Here's how the part is built. I have some questions about the finished solid (model axes, mm). Round coordinates to 2 decimals unless told otherwise and drop trailing zeros. Loops run counter-clockwise (first coordinate to the right, second up) from the corner with the lowest first, then second, coordinate; pieces in that order, holes last. Notation, with made-up numbers: M 68.25,49.25 L 124.25,49.25 A19 ccw 124.25,60.25 Z; hole C 18.25,83 d6. An arc over 180 degrees is marked long. One line per question, with ' | ' between items. Start each with the question number.
```python
from build123d import *

# Parameters (mm, degrees)
BOSS_EXTRUDE1_DEPTH = 2.0574
FILLET1_R           = 1.0287


with BuildPart() as part:
    # Sketch1 → Boss-Extrude1 (new body)
    with BuildSketch(Plane(origin=(0, 0, 0), x_dir=(1, 0, 0), z_dir=(0, 1, 0))):
        Polygon((0, 0), (404.576362049, 0), (316.588181024, 152.4), (87.988181024, 152.4), align=None)
    extrude(amount=BOSS_EXTRUDE1_DEPTH)

    # Fillet1
    fillet1_edges = [part.edges().sort_by_distance(p)[0] for p in [
        (202.288181024, 2.0574, 0),
    ]]
    fillet(fillet1_edges, radius=FILLET1_R)


solid = part.part
```
1) Please list where these lines run through material, in increasing order: L1, parallel to Z at x = 198, y = 1.25; L2, parallel to Z at x = 127.5, y = 1.35; L3, parallel to X at y = 1.5, z = -121.5. Write a range as from..to.
2) I'm going to push a flat-ended pin straight in: pin 1 Ø1 at (y, z) = (1, -68.5) entering from -X. Where does the tip first touch, or does it pass through?
3) Imagine slicing it at B-B (x = 56). Write out the boundary of the cut face in (y, z).
4) Imagine slicing it at C-C (z = -104.5). Write out the boundary of the cut face in (x, y), then the cut area to 3 significant figures.
5) Imagine slicing it at D-D (x = 358.5). Write out the boundary of the cut face in (y, z).
6) Imagine slicing it at A-A (y = 0.6). Write out the boundary of the cut face in (x, z), then the cut area to 3 significant figures.
Results are:
1) L1: -152.4..-0.02 | L2: -152.4..-0.05 | L3: 70.15..334.43
2) pin 1: x = 39.26
3) outline: M 0,-96.99 L 2.06,-96.99 L 2.06,-1.03 A1.03 ccw 1.03,0 L 0,0 Z
4) outline: M 60.33,0 L 344.24,0 L 344.24,2.06 L 60.33,2.06 Z | area: 584 mm²
5) outline: M 0,-79.81 L 2.06,-79.81 L 2.06,-1.03 A1.03 ccw 1.03,0 L 0,0 Z
6) outline: M 0,0 L 87.99,-152.4 L 316.59,-152.4 L 404.58,0 Z | area: 48,200 mm²
